Autodesk Inventor part; units mm, degrees
ref_plane "Work Plane1" through (104.775, 0, 0) normal (0, 0, -1) x (1, 0, 0)
ref_plane "YZ Plane" through (0, 0, 0) normal (1, 0, 0) x (0, 1, 0)
ref_plane "XZ Plane" through (0, 0, 0) normal (0, 1, 0) x (-1, 0, 0)
sketch "Sketch1" plane through (0, 0, 0) normal (0, 0, 1) x (1, 0, 0)
  line L0 (25, 0) -> (25, 1.5)
  line L1 (25, 1.5) -> (3.36, 1.5)
  line L2 (3.36, 1.5) -> (3.0533, 1.5)
  line L3 (0, 2.77) -> (0, 1.1547)
  line L4 (0, 1.1547) -> (1.1, 1.1547)
  line L5 (1.1, 1.1547) -> (1.7667, 0)
  line L6 (1.7667, 0) -> (25, 0)
  line L7 (0, 2.77) -> (0.59, 2.77)
  line L8 (0.59, 2.77) -> (1.86, 1.5)
  line L9 (3.0533, 1.5) -> (1.86, 1.5)
  line L10 (3.36, 1.5) -> (1.86, 1.5) construction
  line L11 (1.86, 1.5) -> (1.86, 1.5)
  line L12 (-25.4, 0) -> (152.4, 0)
  line L13 (0, -2.1133) -> (0, 12.6797)
  dimension "d0" = 25
  dimension "d1" = 21.64
  dimension "d2" = 1.1
  dimension "d3" = 3
  dimension "d6" = 1.86
  dimension "d7" = 45
  dimension "d8" = 2.3094
  dimension "d9" = 60
  dimension "d10" = 5.54
  dimension "d11" = 3
  dimension "d12" = 0.3067
revolve "Body" add sketch "Sketch1" angle 360 about axis through (1.7667, 0, 0) along (1, 0, 0) contours L6 L5 L4 L3 L7 L8 L9 L2 L1 L0
sketch "Sketch2" plane through (0, 0, 0) normal (-1, 0, 0) x (0, 0, 1)
  circle A0 centre (0, 0) radius 1.1547
  line L0 (0, -6.4055) -> (0, 6.4055)
  line L1 (-6.4055, 0) -> (6.4055, 0)
  line L2 (1.1547, 0) -> (0.5774, -1)
  line L3 (0.5774, -1) -> (-0.5774, -1)
  line L4 (-0.5774, -1) -> (-1.1547, 0)
  line L5 (-1.1547, 0) -> (-0.5774, 1)
  line L6 (-0.5774, 1) -> (0.5774, 1)
  line L7 (0.5774, 1) -> (1.1547, 0)
  point P0 (0, 1.1547)
extrude "Slot" add sketch "Sketch2" against normal up to next contours L7 A0 | A0 L2 | L6 L0 A0 | A0 L0 L3 | L0 L6 A0 | A0 L3 L0 | L4 A0 | A0 L5
thread "Thread"
chamfer "Chamfer1" distance 0.3067 distance2 0.3067 1 edges at (25, -1.5, 0) measured on face at (25, 0.0871, 0.3876)
ref_plane "Work Plane1" through (104.775, 0, 0) normal (0, 0, -1) x (1, 0, 0)
equation "\"d15\" = GEL"
equation "\"d17\" = -0.5 * SPD + 0.5 * GD"
equation "\"d18\" = GUL"
equation "\"d0\" = NLG"
equation "\"d1\" = GEL"
equation "\"d2\" = INTI"
equation "\"d3\" = GD"
equation "\"d6\" = KOH"
equation "\"d7\" = 0.5 * SEWI"
equation "\"d8\" = 1.1547 * SW"
equation "\"d10\" = KOD"
equation "\"d11\" = BDM"
equation "\"d12\" = GAL"
equation "\"NLG\" = 25"
equation "\"INTI\" = 1.1"
equation "\"GEL\" = 21.64"
equation "\"GAL\" = 0.61345 * PTC"
equation "\"KOH\" = 1.86"
equation "\"KOD\" = 5.54"
equation "\"GUL\" = 0.61345 * PTC"
equation "\"SPD\" = NND - 1.2269 * PTC"
equation "\"BDM\" = NND"
equation "\"GD\" = NND"
equation "\"SEWI\" = 90deg"
equation "\"SW\" = 2"
equation "\"TOA\" = 30deg"
equation "\"GD1\" = THREADDIA - 1.2269 * PTC"
equation "\"EPV\" = 3.36"
equation "\"THREADDIA\" = 3"
equation "\"PTC\" = 0.5"
equation "\"NND\" = 3"
equation "\"E0\" = 2.31"
properties part number "ISO 10642  - M3  x  25" material "Steel"
Can you work these out from the model? Positions are in its coordinate system, mm. A direction names the side the tool comes from. Coordinates: 2 decimals unless noted, no trailing zeros. Order: outer loops, then holes, each group sorted by start corner. A loop starts at its lowest first (then second) coordinate and runs counter-clockwise, first axis right, second up.
1. I need wall thicknesses on line 1 (Z direction, x = 16, y = 0.95); line 2 (X direction, y = 0.35, z = -0.9); line 3 (Y direction, x = 3.5, z = -0.25). Which ranges of each line are inside material? Lowest first, please.
2. I'm going to push flat-ended pins straight in: pin 1 (1.5 mm diameter, centred on x = 6.5, y = 0.5, fed in from -Z); pin 2 (1 mm diameter, centred on x = 22, y = 0, fed in from +Z); pin 3 (1 mm diameter, centred on x = 19.5, z = -0.5, fed in from +Y); pin 4 (1 mm diameter, centred on y = 1.5, z = 0, fed in from -X). Where does each tip first touch, or does it pass through?
3. Thinking about a two-plate mould opening in Z: for faces 1 (the face through (13.12, -1.5, -0.07)), 2 (the face through (0.59, -0.51, -0.86)), 3 (the face through (25, 0, 0)), which applies, +Z half, -Z half, draft (parallel to the pull), parting line (faces both ways), or undercut?
4. For faces 4 (the face through (0.299, 2.642, 0.832)), 5 (the face through (1, 1, 0)), which set-ups out of +Z, -Z, +X, -X, +Y, -Y let a thin tool reach every point of the face, with its end or its side?
5. If we section it at A-A (x = 23): Please give me the cut outline in (y, z).
Entries:
1. line 1: z = -1.16 to 1.16
1. line 2: x = 1.21 to 25
1. line 3: y = -1.48 to 1.48
2. pin 1: stops at z = -1.5
2. pin 2: stops at z = 1.5
2. pin 3: stops at y = 1.5
2. pin 4: stops at x = 0
3. face 1: parting line
3. face 2: undercut
3. face 3: draft
4. face 4: +X, -X
4. face 5: -X
5. outline: circle Ø3 at (0, 0)
